The listing builds one solid part. Answer for the finished solid, in the listing's coordinates (mm). A direction names the side the tool comes from. Coordinates: 2 decimals unless noted, no trailing zeros. Write each loop counter-clockwise with the first axis right and the second up, starting at its lowest first coordinate (ties: lowest second). Pieces come first, ordered by that corner, then holes.
(1) The part is cut by section B-B on x = 7.5. Determine the outline of the cut face in (y, z), plus the area to 3 significant figures.
(2) The part is cut by section C-C on y = -44.5. Determine the outline of the cut face in (x, z) (3 decimals).
(3) Which of the six approach directions +Z, -Z, +X, -X, +Y, -Y give full straight-line access (tool end or side, diameter ignored) to faces 1 (the cylindrical face through (-14.302, -37.567, 24.895)), 2 (the cylindrical face through (56.91, -38.63, 28.07))?
(4) Straight lines are drawn through the part: line 1 (Z direction, x = -8.5, y = -45); line 2 (X direction, y = -67, z = 18); line 3 (X direction, y = -14.5, z = 26). For each, find the intervals that lie inside material, in ascending order.
(5) The part is cut by section A-A on z = 19.25. Determine the outline of the cut face in (x, y), plus the area to 3 significant figures.
(6) For a pull along Z with two mould halves and no side action, classify faces 3 (the flat face through (19, -38, 29.025)), 4 (the flat face through (19, -38, 3.625)), 5 (the flat face through (54.643, -38, 16)) as +Z half, -Z half, draft (parallel to the pull), parting line (faces both ways), or undercut.
from build123d import *

# Parameters (mm, degrees)
F0_W     = 76.2
F0_H     = 25.4
F1_DEPTH = 76.2
F2_T     = -3.175
F3_R     = 3.175


with BuildPart() as f1:
    # F0 (on Front) → F1 (new body)
    with BuildSketch(Plane.XZ):
        with Locations((19.7176617778, 16.3246961311)):
            Rectangle(F0_W, F0_H)
    extrude(amount=F1_DEPTH)

    # F2
    f2_openings = [f1.faces().sort_by_distance(p)[0] for p in [
        (19.717662, -76.2, 16.324696),
        (19.717662, 0, 16.324696),
    ]]
    offset(amount=F2_T, openings=f2_openings)

    # F3
    f3_edges = [f1.edges().sort_by_distance(p)[0] for p in [
        (-18.382338, -38.1, 29.024696),
        (-15.207338, -38.1, 25.849696),
        (-15.207338, -38.1, 6.799696),
        (54.642662, -38.1, 6.799696),
        (54.642662, -38.1, 25.849696),
        (-18.382338, -38.1, 3.624696),
        (57.817662, -38.1, 29.024696),
        (57.817662, -38.1, 3.624696),
    ]]
    fillet(f3_edges, radius=F3_R)


solid = f1.part
Model answer:
1. outline: (-76.2, 3.62) - (0, 3.62) - (0, 6.8) - (-76.2, 6.8) - close; (-76.2, 25.85) - (0, 25.85) - (0, 29.02) - (-76.2, 29.02) - close
1. area: 484 mm2
2. outline: (-18.382, 6.8) arc R3.175 ccw to (-15.207, 3.625) - (54.643, 3.625) arc R3.175 ccw to (57.818, 6.8) - (57.818, 25.85) arc R3.175 ccw to (54.643, 29.025) - (-15.207, 29.025) arc R3.175 ccw to (-18.382, 25.85) - close; hole (-15.207, 9.975) arc R3.175 ccw to (-12.032, 6.8) - (51.468, 6.8) arc R3.175 ccw to (54.643, 9.975) - (54.643, 22.675) arc R3.175 ccw to (51.468, 25.85) - (-12.032, 25.85) arc R3.175 ccw to (-15.207, 22.675) - close
3. face 1: +Y, -Y
3. face 2: +Z, +X, +Y, -Y
4. line 1: z = 3.62 to 6.8, 25.85 to 29.02
4. line 2: x = -18.38 to -15.21, 54.64 to 57.82
4. line 3: x = -18.38 to 57.81
5. outline: (-18.38, -76.2) - (-15.21, -76.2) - (-15.21, 0) - (-18.38, 0) - close; (54.64, -76.2) - (57.82, -76.2) - (57.82, 0) - (54.64, 0) - close
5. area: 484 mm2
6. face 3: +Z half
6. face 4: -Z half
6. face 5: undercut
